Geometry: see drawing. Coordinates: mm, zero at the bounding-box minimum. A direction names the side the tool comes from. Give positions to 0.01 mm unless a question says otherwise; leave off trailing zeros. Order: outer loops, then holes, each group sorted by start corner. A loop starts at its lowest first (then second) coordinate and runs counter-clockwise, first axis right, second up. Notation, with made-up numbers: (30.5, 35.25) - (42.5, 35.25) arc R9 cw to (42.5, 42.25) - close; hole circle Ø5 at (46.25, -32.75). An arc over 180 degrees is marked (long way). Write each question's results on one line, items separated by ' | '. Start each with the question number.
Item 1: Mould query, pull axis Z, two halves, no side actions, for the marked faces 1, 2, 3 and 4. Classes: released by +Z, released by -Z, zero draft, split by the parting line, or undercut.
Item 2: Line query: line 1 along Z through (x, y) = (36, 11.75); line 2 along X through (y, z) = (11.25, 14); line 3 along Y through (x, z) = (19.5, 14.75). Output: solid intervals per line, ascending.
Item 3: Set-up query: the marked faces 5, 6, 7 and 8. Return all of +Z, -Z, +X, -X, +Y, -Y with unobstructed straight access to the full face (end or side cutting, diameter ignored); none if empty.
Item 4: Section A-A on y = 2.5. Output: boundary loops of the cut face in (x, z).
Item 5: Section D-D on y = 14.75. Output: boundary loops of the cut face in (x, z).
Item 6: Contact query for flat-ended pins moving along their axis: pin 1 Ø1.5 at (x, z) = (17.5, 21.5) entering from +Y; pin 2 Ø10 at (x, y) = (18.5, 19) entering from -Z; pin 3 Ø11 at (y, z) = (20.5, 4.5) entering from +X; pin 4 Ø4 at (y, z) = (19.5, 18.5) entering from +X. Output: stop coordinate, or through.
Item 7: Section B-B on z = 17.75. Output: boundary loops of the cut face in (x, y), and give its area (3 significant figures).
Item 8: Section C-C on x = 27. Output: boundary loops of the cut face in (y, z).
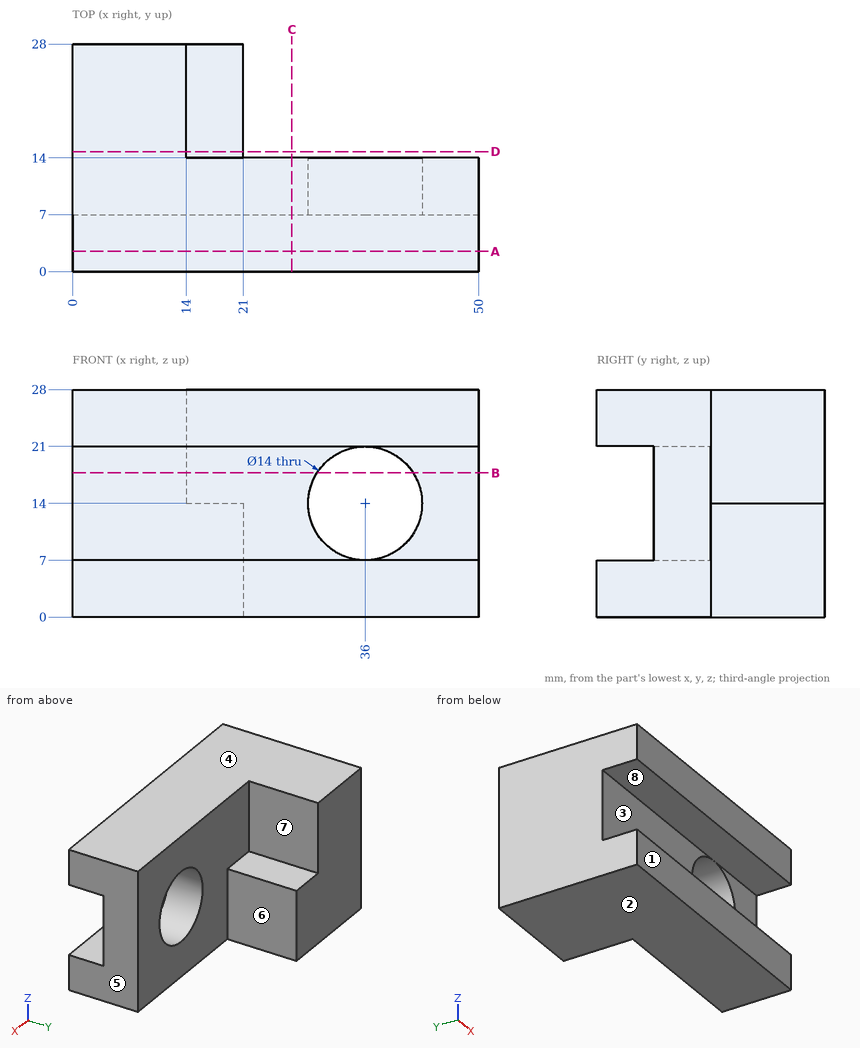
Evaluation:
1) face 1: zero draft | face 2: released by -Z | face 3: undercut | face 4: released by +Z
2) line 1: z = 0 to 7, 21 to 28 | line 2: x = 0 to 29, 43 to 50 | line 3: y = 7 to 14
3) face 5: +Z, -Z, +X, +Y, -Y | face 6: +Z, -Z, +X, +Y | face 7: +Z, +X, +Y | face 8: +X, -X, -Y
4) outline: (0, 0) - (50, 0) - (50, 7) - (0, 7) - close; (0, 21) - (50, 21) - (50, 28) - (0, 28) - close
5) outline: (0, 0) - (21, 0) - (21, 14) - (14, 14) - (14, 28) - (0, 28) - close
6) pin 1: stops at y = 14 | pin 2: stops at z = 0 | pin 3: stops at x = 21 | pin 4: stops at x = 14
7) outline: (0, 7) - (30.09, 7) - (30.09, 14) - (14, 14) - (14, 28) - (0, 28) - close; (41.91, 7) - (50, 7) - (50, 14) - (41.91, 14) - close | area: 463 mm^2
8) outline: (0, 0) - (14, 0) - (14, 28) - (0, 28) - (0, 21) - (7, 21) - (7, 7) - (0, 7) - close
